For this review, take the finished solid that the model builds, in its own axes (mm). A direction names the side the tool comes from. Give positions to 0.01 mm unless a question says otherwise; leave off trailing zeros. Loops run counter-clockwise (first coordinate to the right, second up) from the corner with the lowest first, then second, coordinate; pieces in that order, holes last. Notation, with made-up numbers: (33.5, 37) - (63.5, 37) arc R35 cw to (63.5, 70) - close; hole circle Ø5 at (78.5, 29.5). An arc over 180 degrees is marked (long way). Answer in a Markdown table with one row per item.
Autodesk Inventor part; units mm, degrees
ref_plane "YZ Plane" through (0, 0, 0) normal (1, 0, 0) x (0, 1, 0)
ref_plane "XZ Plane" through (0, 0, 0) normal (0, 1, 0) x (-1, 0, 0)
ref_plane "XY Plane" through (0, 0, 0) normal (0, 0, 1) x (1, 0, 0)
sketch "Sketch1" plane through (0, 0, 0) normal (0, 0, 1) x (1, 0, 0)
  line L0 (-35.7, -23.5) -> (35.7, -23.5)
  line L1 (35.7, -23.5) -> (35.7, 23.5)
  line L2 (35.7, 23.5) -> (-35.7, 23.5)
  line L3 (-35.7, 23.5) -> (-35.7, -23.5)
  line L4 (-35.7, -23.5) -> (35.7, 23.5) construction
  line L5 (35.7, -23.5) -> (-35.7, 23.5) construction
  point P0 (0, 0)
  dimension "d0" = 47
  dimension "d1" = 71.4
extrude "Extrusion1" add sketch "Sketch1" along normal blind 1.6
sketch "Sketch2" plane through (0, 0, 0) normal (0, 0, -1) x (-1, 0, 0)
  line L0 (35.7, -23.5) -> (-35.7, -23.5)
  line L1 (35.7, -23.5) -> (-35.7, -23.5)
  line L2 (15.1, -23.5) -> (22.3, -23.5)
  line L3 (22.3, -23.5) -> (22.3, -16.5)
  line L4 (22.3, -16.5) -> (15.1, -16.5)
  line L5 (15.1, -16.5) -> (15.1, -23.5)
  line L6 (-35.7, -23.5) -> (-35.7, 23.5)
  point P0 (0, 0)
  dimension "d4" = 50.8
  dimension "d5" = 7.2
  dimension "d6" = 7
extrude "Extrusion2" cut sketch "Sketch2" against normal through all
sketch "Sketch3" plane through (0, 0, 0) normal (0, 0, -1) x (-1, 0, 0)
  circle A0 centre (30.7, 18.5) radius 1.375
  circle A1 centre (-30.7, -5.5) radius 1.375
  circle A2 centre (-30.7, 18.5) radius 1.375
  line L0 (35.7, 23.5) -> (35.7, -23.5)
  line L1 (-35.7, 23.5) -> (35.7, 23.5)
  line L2 (-35.7, -23.5) -> (-35.7, 23.5)
  line L3 (15.1, -23.5) -> (-35.7, -23.5)
  circle A3 centre (18.7, -5.5) radius 1.375
  line L4 (15.1, -23.5) -> (15.1, -16.5)
  line L5 (22.3, -16.5) -> (22.3, -23.5)
  point P0 (0, 0)
  dimension "d9" = 2.75
  dimension "d10" = 2.75
  dimension "d11" = 2.75
  dimension "d12" = 5
  dimension "d13" = 5
  dimension "d14" = 5
  dimension "d15" = 5
  dimension "d16" = 5
  dimension "d17" = 18
  dimension "d20" = 2.75
  dimension "d21" = 0
  dimension "d22" = 7.2
  dimension "d23" = 3.6
extrude "Extrusion3" cut sketch "Sketch3" against normal through all
fillet "Fillet1" radius 1 8 edges at (35.7, 23.5, 0.8) (-35.7, 23.5, 0.8) (-35.7, -23.5, 0.8) (-15.1, -23.5, 0.8) (-22.3, -23.5, 0.8) (-15.1, -16.5, 0.8) (-22.3, -16.5, 0.8) (35.7, -23.5, 0.8)
sketch "PWR_PCBA_OUTLINE" plane through (0, 0, 0) normal (0, 0, -1) x (-1, 0, 0)
  line L0 (16.1, -16.5) -> (21.3, -16.5)
  arc A0 (16.1, -16.5) -> (15.1, -17.5) centre (16.1, -17.5) ccw
  line L1 (15.1, -22.5) -> (15.1, -17.5)
  arc A1 (14.1, -23.5) -> (15.1, -22.5) centre (14.1, -22.5) ccw
  line L2 (14.1, -23.5) -> (-34.7, -23.5)
  arc A2 (-35.7, -22.5) -> (-34.7, -23.5) centre (-34.7, -22.5) ccw
  line L3 (-35.7, -22.5) -> (-35.7, 22.5)
  arc A3 (-34.7, 23.5) -> (-35.7, 22.5) centre (-34.7, 22.5) ccw
  line L4 (-34.7, 23.5) -> (34.7, 23.5)
  arc A4 (35.7, 22.5) -> (34.7, 23.5) centre (34.7, 22.5) ccw
  line L5 (35.7, 22.5) -> (35.7, -22.5)
  arc A5 (34.7, -23.5) -> (35.7, -22.5) centre (34.7, -22.5) ccw
  line L6 (34.7, -23.5) -> (23.3, -23.5)
  arc A6 (22.3, -22.5) -> (23.3, -23.5) centre (23.3, -22.5) ccw
  line L7 (22.3, -17.5) -> (22.3, -22.5)
  arc A7 (22.3, -17.5) -> (21.3, -16.5) centre (21.3, -17.5) ccw
  circle A8 centre (12.56, -19.5) radius 0.7937
  circle A9 centre (-33.16, -19.5) radius 0.7938
  line L8 (28.691, 15) -> (37.2, 15)
  line L9 (28.691, -10.908) -> (37.2, -10.908)
  line L10 (28.691, -10.908) -> (28.691, -10.4)
  line L11 (28.691, 14.492) -> (28.691, 15)
  line L12 (27.3702, 13.8697) -> (26.9638, 13.8697)
  line L13 (27.3702, 13.623) -> (27.3702, 13.8697)
  line L14 (27.3702, 13.623) -> (27.3702, 13.329)
  line L15 (27.3702, 13.0823) -> (27.3702, 13.329)
  line L16 (26.9638, 13.0823) -> (27.3702, 13.0823)
  line L17 (26.9638, 13.329) -> (26.9638, 13.0823)
  line L18 (26.9638, 13.329) -> (26.9638, 13.623)
  line L19 (26.9638, 13.8697) -> (26.9638, 13.623)
  line L20 (24.8302, -9.237) -> (24.8302, -9.531)
  line L21 (24.8302, -9.237) -> (24.8302, -8.9903)
  line L22 (24.8302, -8.9903) -> (24.4238, -8.9903)
  line L23 (24.4238, -8.9903) -> (24.4238, -9.237)
  line L24 (24.4238, -9.531) -> (24.4238, -9.237)
  line L25 (24.4238, -9.531) -> (24.4238, -9.7777)
  line L26 (24.4238, -9.7777) -> (24.8302, -9.7777)
  line L27 (24.8302, -9.7777) -> (24.8302, -9.531)
  circle A10 centre (24.627, -9.384) radius 0.2032
  circle A11 centre (27.167, 13.476) radius 0.2032
  circle A12 centre (18.7, -5.5) radius 1.375
  circle A13 centre (30.7, 18.5) radius 1.375
  circle A14 centre (-30.7, 18.5) radius 1.375
  circle A15 centre (-30.7, -5.5) radius 1.375
  circle A16 centre (-33.16, -13.5) radius 0.7938
  circle A17 centre (12.56, -13.5) radius 0.7937
  point P0 (0, 0)
  dimension "d29" = 0.7874
  dimension "d30" = 0.3937
  dimension "d31" = 0.3937
  dimension "d32" = 0.7874
equation "\"d10\" = d9"
equation "\"d11\" = d9"
equation "\"d13\" = d12"
equation "\"d14\" = d12"
equation "\"d15\" = d12"
equation "\"d16\" = d12"
equation "\"d20\" = d9"
equation "\"d23\" = 0.5 * d22"
equation "\"d30\" = 0.5 * d29"
equation "\"d31\" = 0.5 * d32"
properties part number "IO_HEADER_PCB"
1. We need section D-D, the plane x = 30.7. Give the boundary of the cut face in (y, z) (3 decimals).
Values:
| item | result |
|---|---|
| outline | (-23.5, 0) - (-6.875, 0) - (-6.875, 1.6) - (-23.5, 1.6) - close; (-4.125, 0) - (17.125, 0) - (17.125, 1.6) - (-4.125, 1.6) - close; (19.875, 0) - (23.5, 0) - (23.5, 1.6) - (19.875, 1.6) - close |
2. We need section B-B, the plane y = -5.5. Give the boundary of the cut face in (x, z) (3 decimals).
Values:
| item | result |
|---|---|
| outline | (-35.7, 0) - (-20.075, 0) - (-20.075, 1.6) - (-35.7, 1.6) - close; (-17.325, 0) - (29.325, 0) - (29.325, 1.6) - (-17.325, 1.6) - close; (32.075, 0) - (35.7, 0) - (35.7, 1.6) - (32.075, 1.6) - close |
3. Wall thickness on line 1 (Y direction, x = 30.7, z = 0.85) (3 decimals); line 2 (X direction, y = -21, z = 0.4); line 3 (X direction, y = -4.5, z = 0.3): over which ranges is each line inside the solid? List them lowest first. Write a range as [from, to].
Values:
| item | result |
|---|---|
| line 1 | y = [-23.5, -6.875], [-4.125, 17.125], [19.875, 23.5] |
| line 2 | x = [-35.7, -22.3], [-15.1, 35.7] |
| line 3 | x = [-35.7, -19.64], [-17.76, 29.76], [31.64, 35.7] |
4. For faces 4 (the face through (-29, -23.5, 1)), 5 (the face through (-15.1, -20, 1)), list the 3-axis set-ups (+Z, -Z, +X, -X, +Y, -Y) from which the entire face can be reached by the end or side of a thin tool; tool diameter is ignored.
Values:
| item | result |
|---|---|
| face 4 | +Z, -Z, +X, -X, -Y |
| face 5 | +Z, -Z, -Y |
5. Clearance check with flat-ended pins moving along their axes: pin 1 (6 mm diameter, centred on x = -9, y = -5.5, fed in from -Z); pin 2 (2.5 mm diameter, centred on x = -30.7, y = 18.5, fed in from +Z). State where each tip first meets the part, or that it passes through.
Values:
| item | result |
|---|---|
| pin 1 | stops at z = 0 |
| pin 2 | passes through |
6. Mouldability with a two-part tool opening along X and no side actions: class faces 1 (the face through (35.7, 0, 1)), 2 (the face through (29.388, -5.087, 0.789)), 3 (the face through (10, -23.5, 1)) as released by +X, released by -X, zero draft, split by the parting line, or undercut.
Values:
| item | result |
|---|---|
| face 1 | released by +X |
| face 2 | undercut |
| face 3 | zero draft |
7. We need section A-A, the plane x = -30.7. Give the boundary of the cut face in (y, z) (3 decimals).
Values:
| item | result |
|---|---|
| outline | (-23.5, 0) - (17.125, 0) - (17.125, 1.6) - (-23.5, 1.6) - close; (19.875, 0) - (23.5, 0) - (23.5, 1.6) - (19.875, 1.6) - close |
8. We need section C-C, the plane z = 0.8. Give the boundary of the cut face in (x, y) (3 decimals).
Values:
| item | result |
|---|---|
| outline | (-35.7, -22.5) arc R1 ccw to (-34.7, -23.5) - (-23.3, -23.5) arc R1 ccw to (-22.3, -22.5) - (-22.3, -17.5) arc R1 cw to (-21.3, -16.5) - (-16.1, -16.5) arc R1 cw to (-15.1, -17.5) - (-15.1, -22.5) arc R1 ccw to (-14.1, -23.5) - (34.7, -23.5) arc R1 ccw to (35.7, -22.5) - (35.7, 22.5) arc R1 ccw to (34.7, 23.5) - (-34.7, 23.5) arc R1 ccw to (-35.7, 22.5) - close; hole circle Ø2.75 at (-30.7, 18.5); hole circle Ø2.75 at (-18.7, -5.5); hole circle Ø2.75 at (30.7, -5.5); hole circle Ø2.75 at (30.7, 18.5) |
